from build123d import *

# Parameters (mm, degrees)
SKETCH_R             = 80
SKETCH_R_2           = 15
SKETCH_R_3           = 1
PAD_DEPTH            = 3
SKETCH001_R          = 30
SKETCH001_R_2        = 27
PAD001_DEPTH         = 45
SKETCH002_R          = 6
PAD002_DEPTH         = 45
SKETCH004_R          = 1.6
POCKET_DEPTH         = 45.001
SKETCH003_R          = 4
POCKET001_DEPTH      = 20
SKETCH005_R          = 1
POCKET002_DEPTH      = 80.001
POCKET002_DEPTH_BACK = -80.001
POCKET003_DEPTH      = 24


with BuildPart() as part:
    # Sketch → Pad (new body)
    with BuildSketch(Plane.XY):
        Circle(SKETCH_R)
        Circle(SKETCH_R_2, mode=Mode.SUBTRACT)
        with Locations((-66.683956, 38.5)):
            Circle(SKETCH_R_3, mode=Mode.SUBTRACT)
        with Locations((66.683956, 38.5)):
            Circle(SKETCH_R_3, mode=Mode.SUBTRACT)
        with Locations((0, -77)):
            Circle(SKETCH_R_3, mode=Mode.SUBTRACT)
        with BuildLine():
            ThreePointArc((-15, 45), (0, 30), (15, 45))
            Line((15, 45), (15, 60))
            ThreePointArc((15, 60), (0, 75), (-15, 60))
            Line((-15, 45), (-15, 60))
        make_face(mode=Mode.SUBTRACT)
        with BuildLine():
            ThreePointArc((-31.471143, -35.490381), (-25.980762, -15), (-46.471143, -9.509619))
            Line((-46.471143, -9.509619), (-59.461524, -17.009619))
            ThreePointArc((-59.461524, -17.009619), (-64.951905, -37.5), (-44.461524, -42.990381))
            Line((-31.471143, -35.490381), (-44.461524, -42.990381))
        make_face(mode=Mode.SUBTRACT)
        with BuildLine():
            ThreePointArc((46.471143, -9.509619), (25.980762, -15), (31.471143, -35.490381))
            Line((31.471143, -35.490381), (44.461524, -42.990381))
            ThreePointArc((44.461524, -42.990381), (64.951905, -37.5), (59.461524, -17.009619))
            Line((46.471143, -9.509619), (59.461524, -17.009619))
        make_face(mode=Mode.SUBTRACT)
    extrude(amount=PAD_DEPTH)

    # Sketch001 → Pad001 (join)
    with BuildSketch(Plane.XY):
        Circle(SKETCH001_R)
        Circle(SKETCH001_R_2, mode=Mode.SUBTRACT)
    extrude(amount=PAD001_DEPTH)

    # Sketch002 → Pad002 (join)
    with BuildSketch(Plane.XY):
        with Locations((-20.78461, 12)):
            Circle(SKETCH002_R)
        with Locations((0, -24)):
            Circle(SKETCH002_R)
        with Locations((20.78461, 12)):
            Circle(SKETCH002_R)
    extrude(amount=PAD002_DEPTH)

    # Sketch004 → Pocket (cut, through all)
    with BuildSketch(Plane.XY):
        with Locations((-20.78461, 12)):
            Circle(SKETCH004_R)
        with Locations((20.78461, 12)):
            Circle(SKETCH004_R)
        with Locations((0, -24)):
            Circle(SKETCH004_R)
    extrude(amount=POCKET_DEPTH, mode=Mode.SUBTRACT)

    # Sketch003 → Pocket001 (cut)
    with BuildSketch(Plane.XY):
        with Locations((-20.78461, 12)):
            Circle(SKETCH003_R)
        with Locations((20.78461, 12)):
            Circle(SKETCH003_R)
        with Locations((0, -24)):
            Circle(SKETCH003_R)
    extrude(amount=POCKET001_DEPTH, mode=Mode.SUBTRACT)

    # Sketch005 → Pocket002 (cut, two sides)
    with BuildSketch(Plane.YZ) as pocket002_sk:
        with Locations((-28, 40)):
            Circle(SKETCH005_R)
    extrude(amount=-POCKET002_DEPTH, mode=Mode.SUBTRACT)
    extrude(pocket002_sk.sketch, amount=-POCKET002_DEPTH_BACK, mode=Mode.SUBTRACT)

    # Sketch006 → Pocket003 (cut)
    with BuildSketch(Plane.XY):
        Polygon((-17.90961, 10.340118), (-17.90961, 13.659882), (-20.78461, 15.319764), (-23.65961, 13.659882), (-23.65961, 10.340118), (-20.78461, 8.680236), align=None)
        Polygon((20.78461, 8.680236), (23.65961, 10.340118), (23.65961, 13.659882), (20.78461, 15.319764), (17.90961, 13.659882), (17.90961, 10.340118), align=None)
        Polygon((2.875, -25.659882), (2.875, -22.340118), (0, -20.680236), (-2.875, -22.340118), (-2.875, -25.659882), (0, -27.319764), align=None)
    extrude(amount=POCKET003_DEPTH, mode=Mode.SUBTRACT)


solid = part.part
Can you work these out from the model? Positions are in its coordinate system, mm. A direction names the side the tool comes from. Round coordinates to 2 decimals unless told otherwise and drop trailing zeros. Write each loop counter-clockwise with the first axis right and the second up, starting at its lowest first coordinate (ties: lowest second). Pieces come first, ordered by that corner, then holes. Notation, with made-up numbers: M -37,72 L 13,72 A22 cw 13,104 Z; hole C 44,0.25 d4. An arc over 180 degrees is marked long. Use a Markdown table: item, result.
Item 1: We'd pull the mould along X, two halves only. Please class faces 5 (the face through (-16, 9, 45)), 6 (the face through (-37.9, -39.2, 1.5)), 7 (the face through (-29.97, 1.32, 23.71)): released by +X, released by -X, zero draft, split by the parting line, or undercut.
Found:
| item | result |
|---|---|
| face 5 | zero draft |
| face 6 | undercut |
| face 7 | split by the parting line |
Item 2: I want a section at C-C (y = 0). List the corners of the cut face in (x, z) for me, and give its area (3 significant figures).
Found:
| item | result |
|---|---|
| outline | M -80,0 L -15,0 L -15,3 L -27,3 L -27,45 L -30,45 L -30,3 L -80,3 Z; M 15,0 L 80,0 L 80,3 L 30,3 L 30,45 L 27,45 L 27,3 L 15,3 Z |
| area | 642 mm2 |
Item 3: If I drill on line 1 along Y through (x, z) = (0, 32.75); line 2 along X through (y, z) = (-13, 34.5); line 3 along X through (y, z) = (15, 6), over which ranges is the centre line in solid material (lowest first)? Write a range as [from, to].
Found:
| item | result |
|---|---|
| line 1 | y = [-30, -25.6], [-22.4, -18], [27, 30] |
| line 2 | x = [-27.04, -23.66], [23.66, 27.04] |
| line 3 | x = [-25.98, -23.43], [-18.14, -15.59], [15.59, 18.14], [23.43, 25.98] |
Item 4: I want a section at A-A (z = 35). List the corners of the cut face in (x, y) for me, and give its area (3 significant figures).
Found:
| item | result |
|---|---|
| outline | C 0,0 d60; hole M -25.64,8.47 A27 ccw -5.48,-26.44 A6 cw long 5.48,-26.44 A27 ccw 25.64,8.47 A6 cw long 20.15,17.97 A27 ccw -20.15,17.97 A6 cw long Z; hole C -20.78,12 d3.2; hole C 0,-24 d3.2; hole C 20.78,12 d3.2 |
| area | 780 mm2 |
Item 5: I want a section at D-D (y = -39.5). List the corners of the cut face in (x, z) for me, and give its area (3 significant figures).
Found:
| item | result |
|---|---|
| outline | M -69.57,0 L -63.57,0 L -63.57,3 L -69.57,3 Z; M -38.42,0 L 38.42,0 L 38.42,3 L -38.42,3 Z; M 63.57,0 L 69.57,0 L 69.57,3 L 63.57,3 Z |
| area | 266 mm2 |
Item 6: I want a section at B-B (x = -37). List the corners of the cut face in (y, z) for me.
Found:
| item | result |
|---|---|
| outline | M -70.93,0 L -38.68,0 L -38.68,3 L -70.93,3 Z; M -7.63,0 L 70.93,0 L 70.93,3 L -7.63,3 Z |
Item 7: Which directions (+Z, -Z, +X, -X, +Y, -Y) give clear straight access to the entire face, cutting with the end or side of a thin tool? Please do faces 1 (the face through (-1, -22, 24)), 2 (the face through (34, 1, 3)), 3 (the face through (0, 75, 1)), 4 (the face through (17, 1, 0)).
Found:
| item | result |
|---|---|
| face 1 | -Z |
| face 2 | +Z |
| face 3 | +Z, -Z |
| face 4 | -Z, +X, -X, +Y, -Y |
Item 8: For pin 1 Ø4 at (x, z) = (9.5, 39.5) entering from +Y; pin 2 Ø2.5 at (y, z) = (53.5, 2) entering from -X; pin 3 Ø2.5 at (y, z) = (54.5, 1.5) entering from +X, each with a flat end and sliding along its axis, tell me the tip position at first contact or that it passes through.
Found:
| item | result |
|---|---|
| pin 1 | stops at y = 29.05 |
| pin 2 | stops at x = -60.58 |
| pin 3 | stops at x = 59.7 |
